Geometry: final body of the model. Coordinates: model frame, mm. A direction names the side the tool comes from. Give positions to 0.01 mm unless a question says otherwise; leave off trailing zeros. Loops run counter-clockwise (first coordinate to the right, second up) from the corner with the lowest first, then second, coordinate; pieces in that order, holes last.
1. Material intervals for line 1 along Z through (x, y) = (-3.75, 6.5); line 2 along Y through (x, z) = (0.5, 97.5), sorted ascending.
2. Section D-D, the plane x = -7. Output: boundary loops of the cut face in (y, z).
3. Section A-A, the plane y = 0. Output: boundary loops of the cut face in (x, z), then the cut area to 3 significant figures.
4. Access query for faces 1 (the face through (-3.905, -0.867, 102.535)), 2 (the face through (0, 0, 105)). Directions: +Z, -Z, +X, -X, +Y, -Y. A direction counts if a zero-diameter tool reaches every point of the face in a straight line with its end or side. Return the directions, or none.
5. Section C-C, the plane z = 31. Output: boundary loops of the cut face in (x, y), then the cut area to 3 significant figures.
6. First-contact query: P1, Ø2, axis at x = -4.5, z = 40.5, coming from the -Y side; P2, Ø1.5, axis at x = 3, z = 86.5, coming from the +Y side; P3, Ø8, axis at y = 2.5, z = 35.5, coming from the +X side. Flat tips, straight axial feed; report the tip coordinate or a pass-through.
from build123d import *

# Parameters (mm, degrees)
F0_R     = 8.5
F1_DEPTH = 4
F2_R     = 5
F3_DEPTH = 100
F4_W     = 4
F4_H     = 5


with BuildPart() as f1:
    # F0 (on Top) → F1 (new body)
    with BuildSketch(Plane.XY):
        Circle(F0_R)
    extrude(amount=F1_DEPTH)

    # F2 (on Top) → F3 (join)
    with BuildSketch(Plane.XY):
        Circle(F2_R)
    extrude(amount=F3_DEPTH)

    # F4 (on Right) → F5 (revolve)
    with BuildSketch(Plane.YZ):
        with Locations((2, 102.5)):
            Rectangle(F4_W, F4_H)
    revolve(axis=Axis((0, 0, 102.5), (0, 0, -1)))


solid = f1.part
Answers below:
1. line 1: z = 0 to 4
1. line 2: y = -4.97 to 4.97
2. outline: (-4.82, 0) - (4.82, 0) - (4.82, 4) - (-4.82, 4) - close
3. outline: (-8.5, 0) - (8.5, 0) - (8.5, 4) - (5, 4) - (5, 100) - (4, 100) - (4, 105) - (-4, 105) - (-4, 100) - (-5, 100) - (-5, 4) - (-8.5, 4) - close
3. area: 1,070 mm2
4. face 1: +Z
4. face 2: +Z, +X, -X, +Y, -Y
5. outline: circle Ø10 at (0, 0)
5. area: 78.5 mm2
6. P1: stops at y = -3.57
6. P2: stops at y = 4.47
6. P3: stops at x = 5
